Autodesk Fusion 360 part; units mm, degrees
sketch "Esquisse1" plane through (0, 0, 0) normal (0, 1, 0) x (1, 0, 0)
  circle A0 centre (0, 0) radius 4
  dimension "d1" = 8
extrude "Extrusion1" add sketch "Esquisse1" along normal blind 15
sketch "Esquisse2" plane through (0, 15, 0) normal (0, 1, 0) x (-1, 0, 0)
  circle A0 centre (0, 0) radius 4
  line L0 (-30.089, 4.9107) -> (29.911, 4.9107)
  line L1 (29.911, 4.9107) -> (29.911, -5.0893)
  line L2 (29.911, -5.0893) -> (-30.089, -5.0893)
  line L3 (-30.089, -5.0893) -> (-30.089, 4.9107)
  point P0 (-0.089, -5.0893)
  dimension "d12" = 60
  dimension "d13" = 10
extrude "Extrusion2" add sketch "Esquisse2" along normal blind 15 contours A0 | L0 L1 L2 L3
sketch "Esquisse5" plane through (0, 0, 0) normal (0, -1, 0) x (1, 0, 0)
  circle A0 centre (0, 0) radius 4
  circle A1 centre (0, 0) radius 2
  dimension "d14" = 4
extrude "Extrusion4" add sketch "Esquisse5" along normal blind 10 contours A1
sketch "Esquisse7" plane through (0, 0, 0) normal (1, 0, 0) x (0, 1, 0)
  line L0 (-10, 2) -> (0, 2)
  line L1 (0, 2) -> (0, 0.5)
  line L2 (0, 0.5) -> (-10, 0.5)
  line L3 (-10, 0.5) -> (-10, 2)
  dimension "d19" = 10
  dimension "d20" = 1.5
extrude "Extrusion5" cut sketch "Esquisse7" along normal blind 3.5 and the other way blind 3
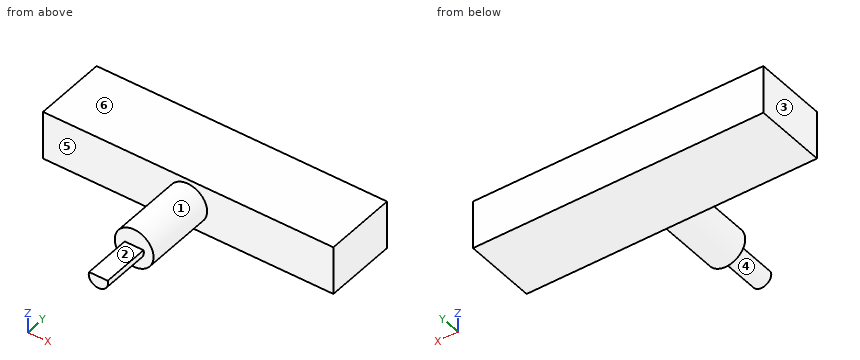
Work out the finished part from the listing and answer in its coordinate system (mm). Face numbers are marked on the shaded views. A direction names the side the tool comes from. Round coordinates to 2 decimals unless told otherwise and drop trailing zeros. Order: outer loops, then holes, each group sorted by start corner. A loop starts at its lowest first (then second) coordinate and runs counter-clockwise, first axis right, second up. Notation, with made-up numbers: M 81,-11 L 116,-11 A8 ccw 116,0 Z; hole C 2.25,-20.5 d5. An arc over 180 degrees is marked long. One line per item, written item: value.
Q1. Find section A-A on x = 0. Write down the section's boundary in (y, z).
Derived:
outline: M -10,-2 L 0,-2 L 0,-4 L 15,-4 L 15,-5.09 L 30,-5.09 L 30,4.91 L 15,4.91 L 15,4 L 0,4 L 0,0.5 L -10,0.5 Z
Q2. Determine the mould class of the marked faces 4, 5 and 6 for opening direction Z: released by +Z, released by -Z, zero draft, split by the parting line, or undercut.
Derived:
face 4: split by the parting line
face 5: zero draft
face 6: released by +Z
Q3. Find section C-C on z = 2.25. Write down the section's boundary in (x, y), then the cut area to 3 significant figures.
Derived:
outline: M -29.91,15 L -3.31,15 L -3.31,0 L 3.31,0 L 3.31,15 L 30.09,15 L 30.09,30 L -29.91,30 Z
area: 999 mm²
Q4. Find section B-B on y = -2. Write down the section's boundary in (x, z), then the cut area to 3 significant figures.
Derived:
outline: M -1.94,0.5 A2 ccw long 1.94,0.5 Z
area: 8.26 mm²
Q5. Flat-ended cylindrical pins translate along their axes: pin 1 (5 mm diameter, centred on x = -11.5, z = 2.5, fed in from -Y); pin 2 (2 mm diameter, centred on y = -1.5, z = -0.5, fed in from -X); pin 3 (3 mm diameter, centred on y = 11.5, z = 2, fed in from -X). Find the tip coordinate at first contact, or state that the pin passes through.
Derived:
pin 1: y = 15
pin 2: x = -2
pin 3: x = -3.97
Q6. For the marked faces 1, 2 and 3, determine the directions among +Z, -Z, +X, -X, +Y, -Y from which every point of the face is accessible in a straight line to the end or side of a thin tool.
Derived:
face 1: -Y
face 2: +Z, +X, -X, -Y
face 3: +Z, -Z, -X, +Y, -Y
Q7. Find section D-D on y = 11. Write down the section's boundary in (x, z), then the cut area to 3 significant figures.
Derived:
outline: C 0,0 d8
area: 50.3 mm²
Q8. Straight lines are drawn through the part: line 1 (X direction, y = -5.5, z = -0.5); line 2 (Y direction, x = 2.5, z = 4.5); line 3 (Y direction, x = -2, z = 1). For each, find the intervals that lie inside material, in ascending order.
Derived:
line 1: -1.94 to 1.94
line 2: 15 to 30
line 3: 0 to 30
